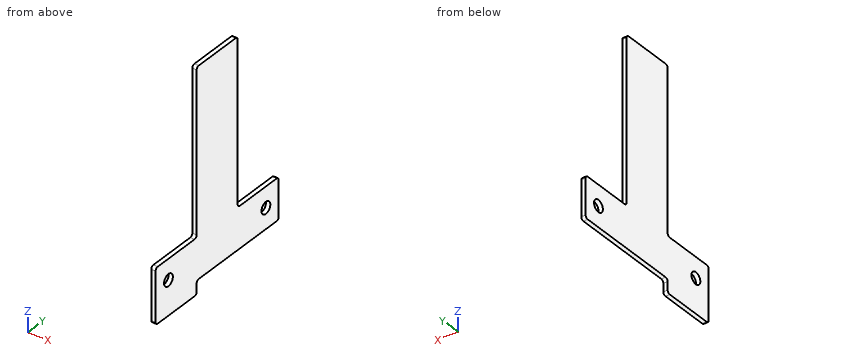
from build123d import *

# Parameters (mm, degrees)
SKETCH1_R           = 2.15
BOSS_EXTRUDE1_DEPTH = 1.5875
FILLET1_R           = 1


with BuildPart() as part:
    # Sketch1 → Boss-Extrude1 (new body)
    with BuildSketch(Plane(origin=(0, 0, 0), x_dir=(0, 0, -1), z_dir=(1, 0, 0))):
        Polygon((-7.5, 30), (7.5, 30), (7.5, -10), (12.5, -10), (12.5, -30), (7.5, -30), (-7.5, -30), (-7.5, -10), (-67.5, -10), (-67.5, 10), (-7.5, 10), align=None)
        with Locations((0, 23.75)):
            Circle(SKETCH1_R, mode=Mode.SUBTRACT)
        with Locations((0, -23.75)):
            Circle(SKETCH1_R, mode=Mode.SUBTRACT)
    extrude(amount=BOSS_EXTRUDE1_DEPTH)

    # Fillet1
    fillet1_edges = [part.edges().sort_by_distance(p)[0] for p in [
        (0.79375, 30, 7.5),
        (0.79375, 30, -7.5),
        (0.79375, -10, -7.5),
        (0.79375, -10, -12.5),
        (0.79375, -30, -12.5),
        (0.79375, -30, 7.5),
        (0.79375, -10, 7.5),
        (0.79375, -10, 67.5),
        (0.79375, 10, 67.5),
        (0.79375, 10, 7.5),
    ]]
    fillet(fillet1_edges, radius=FILLET1_R)


solid = part.part
Design review of the part built by this model. Coordinates are the model's own, in mm. Round coordinates to 2 decimals unless told otherwise and drop trailing zeros. Loops run counter-clockwise (first coordinate to the right, second up) from the corner with the lowest first, then second, coordinate; pieces in that order, holes last. Notation, with made-up numbers: (66.5, 33) - (97.5, 33) arc R15 cw to (97.5, 48) - close; hole circle Ø6 at (-28, -1.5). An arc over 180 degrees is marked (long way). One line per question, with ' | ' between items.
1. Clearance check with flat-ended pins moving along their axes: P1, Ø7, axis at y = 23.75, z = 0, coming from the +X side; P2, Ø0.5, axis at x = 1, y = 5, coming from the -Z side; P3, Ø0.5, axis at x = 0.5, z = 51.5, coming from the -Y side; P4, Ø0.8, axis at x = 0.5, z = 44, coming from the +Y side. State where each tip first meets the part, or that it passes through.
Results are:
P1: stops at x = 1.59 | P2: stops at z = -7.5 | P3: stops at y = -10 | P4: stops at y = 10
2. We need section B-B, the plane z = 0. State the section outline as (x, y) points, and give its area (3 significant figures).
Results are:
outline: (0, -30) - (1.59, -30) - (1.59, -25.9) - (0, -25.9) - close; (0, -21.6) - (1.59, -21.6) - (1.59, 21.6) - (0, 21.6) - close; (0, 25.9) - (1.59, 25.9) - (1.59, 30) - (0, 30) - close | area: 81.6 mm²
3. We need section A-A, the plane y = -23.75. State the section outline as (x, z) points, and give its area (3 significant figures).
Results are:
outline: (0, -12.5) - (1.59, -12.5) - (1.59, -2.15) - (0, -2.15) - close; (0, 2.15) - (1.59, 2.15) - (1.59, 7.5) - (0, 7.5) - close | area: 24.9 mm²
4. For L1, parallel to Y at x = 1.1, z = 0; L2, parallel to Z at x = 0.75, y = -15.5; L3, parallel to Z at x = 0.7, y = 8.5, list the stretches that pass through material, from the lowest coordinate up. Write a range as [from, to].
Results are:
L1: y = [-30, -25.9], [-21.6, 21.6], [25.9, 30] | L2: z = [-12.5, 7.5] | L3: z = [-7.5, 67.5]
5. We need section C-C, the plane x = 1.25. State the section outline as (y, z) points.
Results are:
outline: (-30, -11.5) arc R1 ccw to (-29, -12.5) - (-11, -12.5) arc R1 ccw to (-10, -11.5) - (-10, -8.5) arc R1 cw to (-9, -7.5) - (29, -7.5) arc R1 ccw to (30, -6.5) - (30, 6.5) arc R1 ccw to (29, 7.5) - (11, 7.5) arc R1 cw to (10, 8.5) - (10, 66.5) arc R1 ccw to (9, 67.5) - (-9, 67.5) arc R1 ccw to (-10, 66.5) - (-10, 8.5) arc R1 cw to (-11, 7.5) - (-29, 7.5) arc R1 ccw to (-30, 6.5) - close; hole circle Ø4.3 at (-23.75, 0); hole circle Ø4.3 at (23.75, 0)
6. We need section D-D, the plane y = 23.75. State the section outline as (x, z) points, and give its area (3 significant figures).
Results are:
outline: (0, -7.5) - (1.59, -7.5) - (1.59, -2.15) - (0, -2.15) - close; (0, 2.15) - (1.59, 2.15) - (1.59, 7.5) - (0, 7.5) - close | area: 17.0 mm²
